Work out the finished part from the listing and answer in its coordinate system (mm). Face numbers are marked on the shaded views. A direction names the side the tool comes from. Give positions to 0.01 mm unless a question says otherwise; leave off trailing zeros. Loops run counter-clockwise (first coordinate to the right, second up) from the corner with the lowest first, then second, coordinate; pieces in that order, holes last.
```python
from build123d import *

# Parameters (mm, degrees)
SKETCH1_W           = 500
SKETCH1_H           = 500
BOSS_EXTRUDE1_DEPTH = 500
SKETCH2_R           = 30
SKETCH2_R_2         = 20
BOSS_EXTRUDE2_DEPTH = 1000
SKETCH3_R           = 75
BOSS_EXTRUDE3_DEPTH = 800
SKETCH4_R           = 50
BOSS_EXTRUDE4_DEPTH = 200
SKETCH5_R           = 25
CUT_EXTRUDE1_DEPTH  = 1200
SKETCH6_R           = 15
SKETCH6_R_2         = 10
CUT_EXTRUDE2_DEPTH  = 200


with BuildPart() as part:
    # Sketch1 → Boss-Extrude1 (new body)
    with BuildSketch(Plane(origin=(0, 0, 0), x_dir=(1, 0, 0), z_dir=(0, 1, 0))):
        Rectangle(SKETCH1_W, SKETCH1_H)
    extrude(amount=BOSS_EXTRUDE1_DEPTH)

    # Sketch2 → Boss-Extrude2 (add)
    with BuildSketch(Plane.XZ):
        with Locations(Location((0, 155.7539011, 0), (0, 0, 90))):
            Circle(SKETCH2_R)
        with Locations(Location((-149.221176771, 0, 0), (0, 0, 90))):
            Circle(SKETCH2_R_2)
        with Locations(Location((149.221176771, 0, 0), (0, 0, 90))):
            Circle(SKETCH2_R_2)
        with Locations(Location((0, -111.056313588, 0), (0, 0, 90))):
            Circle(SKETCH2_R)
    extrude(amount=BOSS_EXTRUDE2_DEPTH)

    # Sketch3 → Boss-Extrude3 (add)
    with BuildSketch(Plane(origin=(250, 0, 0), x_dir=(0, 0, -1), z_dir=(1, 0, 0))):
        with Locations((0, 244.080255808)):
            Circle(SKETCH3_R)
    extrude(amount=BOSS_EXTRUDE3_DEPTH)

    # Sketch4 → Boss-Extrude4 (add)
    with BuildSketch(Plane(origin=(1050, 0, 0), x_dir=(0, 0, -1), z_dir=(1, 0, 0))):
        with Locations((0, 244.080255808)):
            Circle(SKETCH4_R)
    extrude(amount=BOSS_EXTRUDE4_DEPTH)

    # Sketch5 → Cut-Extrude1 (cut)
    with BuildSketch(Plane(origin=(1250, 0, 0), x_dir=(0, 0, -1), z_dir=(1, 0, 0))):
        with Locations((0, 244.080255808)):
            Circle(SKETCH5_R)
    extrude(amount=-CUT_EXTRUDE1_DEPTH, mode=Mode.SUBTRACT)

    # Sketch6 → Cut-Extrude2 (cut)
    with BuildSketch(Plane.XZ.offset(1000)):
        with Locations(Location((0, 155.7539011, 0), (0, 0, 270))):
            Circle(SKETCH6_R)
        with Locations(Location((149.221176771, 0, 0), (0, 0, 270))):
            Circle(SKETCH6_R_2)
        with Locations(Location((0, -111.056313588, 0), (0, 0, 270))):
            Circle(SKETCH6_R)
        with Locations(Location((-149.221176771, 0, 0), (0, 0, 270))):
            Circle(SKETCH6_R_2)
    extrude(amount=-CUT_EXTRUDE2_DEPTH, mode=Mode.SUBTRACT)


solid = part.part
```
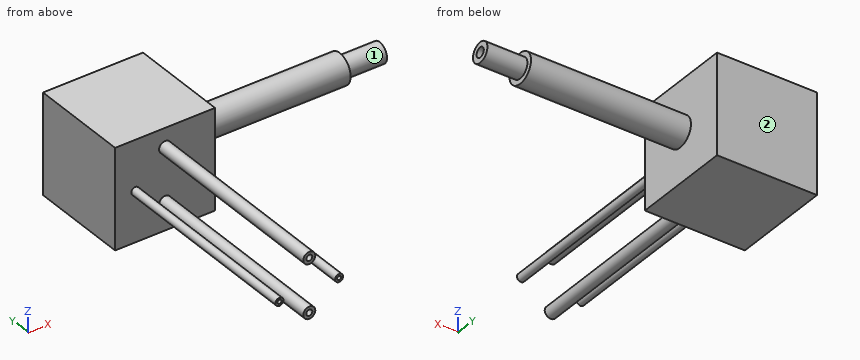
Q1. Consider line 1 along X through (y, z) = (-899, 0); line 2 along X through (y, z) = (313.5, -146); line 3 along Z through (x, y) = (474.5, 251). Determine where each line is inside the solid, lowest interval first.
Q2. Section B-B on x = 202.5 is taken. Give the vertices of the cut face in (y, z), plus the area to 3 significant figures.
Q3. Which of the six approach directions +Z, -Z, +X, -X, +Y, -Y give full straight-line access (tool end or side, diameter ignored) to the marked faces 1 and 2?
Q4. Given pin 1 (6 mm diameter, centred on x = -149.5, z = 1.5, fed in from -Y); pin 2 (2 mm diameter, centred on x = -68.5, z = -49.5, fed in from -Y); pin 3 (8 mm diameter, centred on x = 268, z = 19.5, fed in from +Y), each flat-ended and moving along its own axis, determine where each tip first touches the part or whether it passes through.
Q5. Section A-A on y = -859.5 is taken. Give the vertices of the cut face in (x, z), plus the area to 3 significant figures.
Check result:
1. line 1: x = -169.22 to -159.22, -139.22 to -129.22, 129.22 to 139.22, 159.22 to 169.22
1. line 2: x = -250 to 250
1. line 3: z = -74.68 to -24.02, 24.02 to 74.68
2. outline: (0, -250) - (500, -250) - (500, 250) - (0, 250) - close; hole circle Ø50 at (244.08, 0)
2. area: 248,000 mm2
3. face 1: +X
3. face 2: +Z, -Z, +X, -X, +Y
4. pin 1: stops at y = -800
4. pin 2: stops at y = 0
4. pin 3: stops at y = 317.46
5. outline: circle Ø40 at (-149.22, 0); circle Ø60 at (0, -111.06); circle Ø60 at (0, 155.75); circle Ø40 at (149.22, 0); hole circle Ø20 at (-149.22, 0); hole circle Ø30 at (0, -111.06); hole circle Ø30 at (0, 155.75); hole circle Ø20 at (149.22, 0)
5. area: 6,130 mm2
